The figure shows three views and two pictorial views of one solid part (mm, origin at its lowest corner). Answer the questions. A direction names the side the tool comes from. Round coordinates to 2 decimals unless told otherwise and drop trailing zeros. Order: outer loops, then holes, each group sorted by start corner. A loop starts at its lowest first (then second) coordinate and runs counter-clockwise, first axis right, second up. Notation, with made-up numbers: M -25.75,43 L 10.25,43 A6 ccw 10.25,47 Z; hole C 47,-12.5 d3. An arc over 180 degrees is marked long. Answer as CSV lines item,"result".
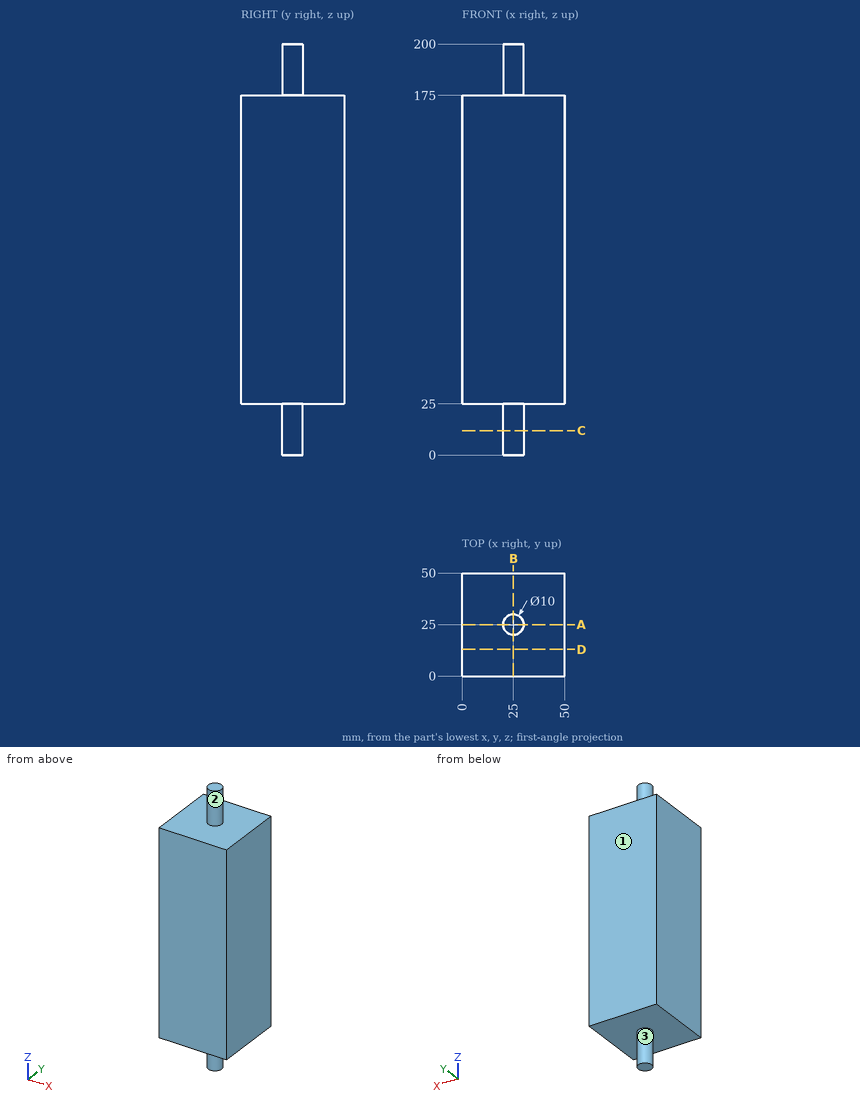
Item 1: Flat-ended cylindrical pins translate along their axes: pin 1 (10 mm diameter, centred on x = 42.5, y = 38.5, fed in from +Z); pin 2 (1.5 mm diameter, centred on x = 40.5, y = 9.5, fed in from -Z); pin 3 (1 mm diameter, centred on y = 42, z = 23.5, fed in from -X); pin 4 (15 mm diameter, centred on x = 22.5, y = 17, fed in from -Z). Find the tip coordinate at first contact, or state that the pin passes through.
Ans:
pin 1,"z = 175"
pin 2,"z = 25"
pin 3,"through"
pin 4,"z = 0"
Item 2: A cutting plane is placed at A-A, the plane y = 25. Determine the outline of the cut face in (x, z).
Ans:
outline,"M 0,25 L 20,25 L 20,0 L 30,0 L 30,25 L 50,25 L 50,175 L 30,175 L 30,200 L 20,200 L 20,175 L 0,175 Z"
Item 3: A cutting plane is placed at C-C, the plane z = 12. Determine the outline of the cut face in (x, y), and give its area (3 significant figures).
Ans:
outline,"C 25,25 d10"
area,"78.5 mm2"
Item 4: A tool of negligible diameter and unlimited length cuts with its end or side. For the marked faces 1, 2 and 3, from which of +Z, -Z, +X, -X, +Y, -Y can it reach the whole face along a straight path? Write none if from no direction.
Ans:
face 1,"+Z, -Z, +X, -X, +Y"
face 2,"+Z"
face 3,"-Z"
Item 5: A cutting plane is placed at D-D, the plane y = 13. Determine the outline of the cut face in (x, z), and give its area (3 significant figures).
Ans:
outline,"M 0,25 L 50,25 L 50,175 L 0,175 Z"
area,"7,500 mm2"
Item 6: Find the intervals of material crossed by probe 1 along Z at (x, y) = (33, 39); probe 2 along X at (y, z) = (23, 185), in increasing order. Write a range as [from, to].
Ans:
probe 1,"[25, 175]"
probe 2,"[20.42, 29.58]"
